Input: dimensioned drawing with shaded views. Units: mm. Origin: part minimum x, y, z. A direction names the side the tool comes from. Coordinates: 2 decimals unless noted, no trailing zeros. Loops run counter-clockwise (first coordinate to the right, second up) from the corner with the lowest first, then second, coordinate; pieces in that order, holes last.
(1) Set-up query: the marked faces 4 and 5. Return all of +Z, -Z, +X, -X, +Y, -Y with unobstructed straight access to the full face (end or side cutting, diameter ignored); none if empty.
(2) Section A-A, the plane x = 15. Return loops of the section in (y, z), then the cut area to 3 significant figures.
(3) Contact query for flat-ended pins moving along their axis: P1, Ø5, axis at y = 19.5, z = 33, coming from the -X side; P2, Ø10, axis at x = 14.5, y = 5.5, coming from the +Z side; P3, Ø2, axis at x = 25.5, z = 46.5, coming from the -Y side. Output: stop coordinate, or through.
(4) Section D-D, the plane y = 21.5. Return loops of the section in (x, z).
(5) Mould query, pull axis X, two halves, no side actions, for the marked faces 1, 2 and 3. Classes: released by +X, released by -X, zero draft, split by the parting line, or undercut.
(6) Section C-C, the plane z = 27.5. Return loops of the section in (x, y), then the cut area to 3 significant figures.
(7) Section B-B, the plane y = 14. Return loops of the section in (x, z).
(8) Line query: L1, parallel to X at y = 26, z = 24; L2, parallel to X at y = 27.5, z = 5.5; L3, parallel to Y at x = 15, z = 21. Output: solid intervals per line, ascending.
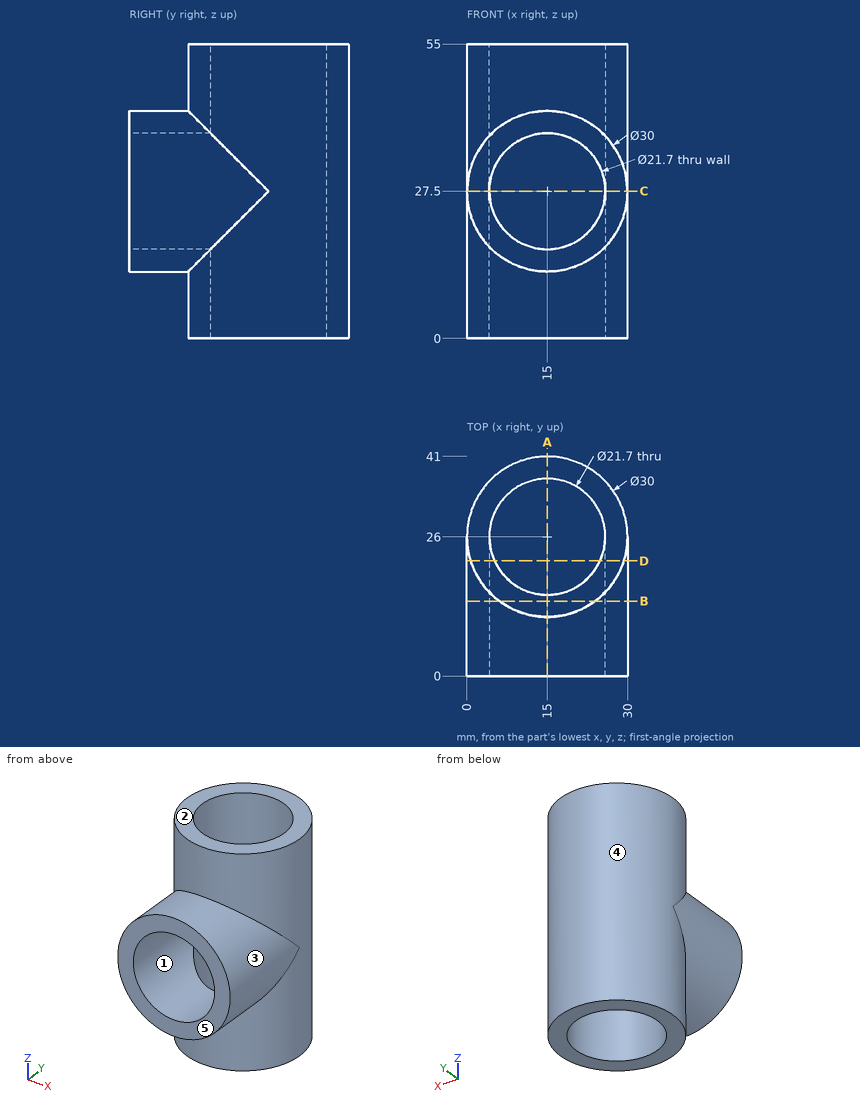
Report:
1. face 4: none
1. face 5: +Z, -Z, +X, -X, -Y
2. outline: (0, 12.5) - (11, 12.5) - (11, 0) - (15.15, 0) - (15.15, 16.65) - (0, 16.65) - close; (0, 38.35) - (15.15, 38.35) - (15.15, 55) - (11, 55) - (11, 42.5) - (0, 42.5) - close; (36.85, 0) - (41, 0) - (41, 55) - (36.85, 55) - close
2. area: 458 mm2
3. P1: stops at x = 0.3
3. P2: stops at z = 42.5
3. P3: stops at y = 14.39
4. outline: (0.69, 0) - (5.13, 0) - (5.13, 23) arc R10.85 cw to (5.13, 32) - (5.13, 55) - (0.69, 55) - (0.69, 32) arc R15 ccw to (0.69, 23) - close; (24.87, 0) - (29.31, 0) - (29.31, 23) arc R15 ccw to (29.31, 32) - (29.31, 55) - (24.87, 55) - (24.87, 32) arc R10.85 cw to (24.87, 23) - close
5. face 1: undercut
5. face 2: zero draft
5. face 3: split by the parting line
6. outline: (0, 0) - (4.15, 0) - (4.15, 26) arc R10.85 cw to (25.85, 26) - (25.85, 0) - (30, 0) - (30, 26) arc R15 ccw to (0, 26) - close
6. area: 384 mm2
7. outline: (6, 0) - (24, 0) - (24, 15.5) arc R15 ccw to (24, 39.5) - (24, 55) - (6, 55) - (6, 39.5) arc R15 ccw to (6, 15.5) - close; hole circle Ø21.7 at (15, 27.5)
8. L1: x = 0 to 4.15, 25.85 to 30
8. L2: x = 0.08 to 4.25, 25.75 to 29.92
8. L3: y = 36.85 to 41
